Geometry: final body of the model. Coordinates: model frame, mm. Give positions to 0.01 mm unless a question says otherwise; leave off trailing zeros. Write each loop counter-clockwise with the first axis right and the second up, starting at its lowest first coordinate (ties: lowest second). Pieces come first, ordered by that corner, then holes.
Q1. Line query: L1, parallel to Y at x = 0, z = 1; L2, parallel to Y at x = -10, z = 0.45; L3, parallel to X at y = 4.5, z = 2.9 (3 decimals). Output: solid intervals per line, ascending.
Q2. Cut plane D-D on y = -24.13. Return the cut outline in (x, z) (3 decimals), plus the area to 3 significant figures.
Q3. Cut plane B-B on x = 17.78. Return the cut outline in (y, z) (3 decimals).
Q4. Cut plane A-A on y = 12.5. Return the cut outline in (x, z) (3 decimals).
Q5. Pin query (flat end, axial travel): pin 1 (2 mm diameter, centred on x = -55.245, y = -24.13, fed in from -Z). Return the tip coordinate at first contact, or that it passes through.
Q6. Cut plane C-C on y = -6.35. Return the cut outline in (x, z) (3 decimals).
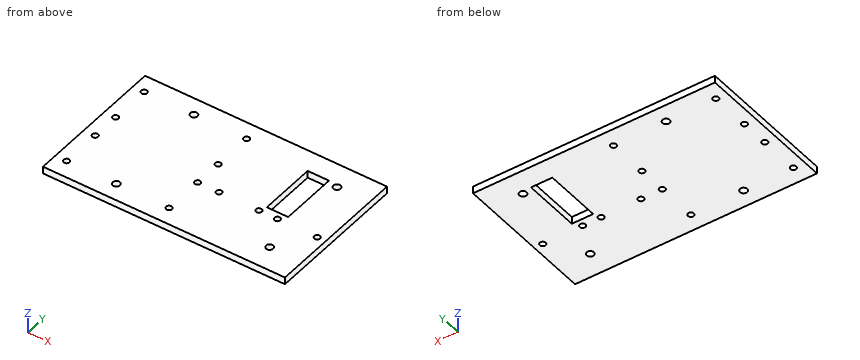
```python
from build123d import *

# Parameters (mm, degrees)
SKETCH1_W               = 95.25
SKETCH1_H               = 63.5
BOSS_EXTRUDE1_DEPTH     = 3.175
SKETCH2_R               = 1.6
CUT_EXTRUDE1_DEPTH      = 58.326117521
CUT_EXTRUDE2_DEPTH      = 58.326117521
CUT_EXTRUDE2_DEPTH_BACK = 58.326117521
SKETCH3_W               = 9.525
SKETCH3_H               = 25.4
SKETCH5_W               = 12.7
SKETCH5_H               = 63.5
BOSS_EXTRUDE2_DEPTH     = 3.175
SKETCH7_R               = 1.3
CUT_EXTRUDE3_DEPTH      = 69.244038201
SKETCH8_R               = 1.29999994
CUT_EXTRUDE4_DEPTH      = 3.175


with BuildPart() as part:
    # Sketch1 → Boss-Extrude1 (new body)
    with BuildSketch(Plane.XY):
        Rectangle(SKETCH1_W, SKETCH1_H)
    extrude(amount=BOSS_EXTRUDE1_DEPTH)

    # Sketch2 → Cut-Extrude1 (cut, through all)
    with BuildSketch(Plane.XY.offset(3.175)):
        with Locations((33.0581, 20.955)):
            Circle(SKETCH2_R)
        with Locations((33.0581, -20.955)):
            Circle(SKETCH2_R)
        with Locations((-33.0581, 24.13)):
            Circle(SKETCH2_R)
        with Locations((-33.0581, -24.13)):
            Circle(SKETCH2_R)
    extrude(amount=-CUT_EXTRUDE1_DEPTH, mode=Mode.SUBTRACT)

    # Sketch3 → Cut-Extrude2 (cut, two sides: drawn at the far end of the back side and taken through both)
    with BuildSketch(Plane.XY.offset(3.175).offset(-CUT_EXTRUDE2_DEPTH_BACK)):
        with Locations((23.8125, 9.525)):
            Rectangle(SKETCH3_W, SKETCH3_H)
    extrude(amount=CUT_EXTRUDE2_DEPTH + CUT_EXTRUDE2_DEPTH_BACK, mode=Mode.SUBTRACT)

    # Sketch5 → Boss-Extrude2 (add)
    with BuildSketch(Plane.XY.offset(3.175)):
        with Locations((-53.975, 0)):
            Rectangle(SKETCH5_W, SKETCH5_H)
    extrude(amount=-BOSS_EXTRUDE2_DEPTH)

    # Sketch7 → Cut-Extrude3 (cut, through all)
    with BuildSketch(Plane.XY.offset(3.175)):
        with Locations((-55.245, 24.13)):
            Circle(SKETCH7_R)
        with Locations((-9.525, 24.13)):
            Circle(SKETCH7_R)
        with Locations((-9.525, 6.35)):
            Circle(SKETCH7_R)
        with Locations((-55.245, 6.35)):
            Circle(SKETCH7_R)
        with Locations((-55.245, -6.35)):
            Circle(SKETCH7_R)
        with Locations((-9.525, -6.35)):
            Circle(SKETCH7_R)
        with Locations((-9.525, -24.13)):
            Circle(SKETCH7_R)
        with Locations((-55.245, -24.13)):
            Circle(SKETCH7_R)
    extrude(amount=-CUT_EXTRUDE3_DEPTH, mode=Mode.SUBTRACT)

    # Sketch8 → Cut-Extrude4 (cut)
    with BuildSketch(Plane.XY.offset(3.175)):
        with Locations((0, -6.35)):
            Circle(SKETCH8_R)
        with Locations((43.815, -6.35)):
            Circle(SKETCH8_R)
        with Locations((17.78, -6.35)):
            Circle(SKETCH8_R)
        with Locations((26.035, -6.35)):
            Circle(SKETCH8_R)
    extrude(amount=-CUT_EXTRUDE4_DEPTH, mode=Mode.SUBTRACT)


solid = part.part
```
Data:
1. L1: y = -31.75 to -7.65, -5.05 to 31.75
1. L2: y = -31.75 to -25.34, -22.92 to -7.56, -5.14 to 5.14, 7.56 to 22.92, 25.34 to 31.75
1. L3: x = -60.325 to 19.05, 28.575 to 47.625
2. outline: (-60.325, 0) - (-56.545, 0) - (-56.545, 3.175) - (-60.325, 3.175) - close; (-53.945, 0) - (-34.658, 0) - (-34.658, 3.175) - (-53.945, 3.175) - close; (-31.458, 0) - (-10.825, 0) - (-10.825, 3.175) - (-31.458, 3.175) - close; (-8.225, 0) - (47.625, 0) - (47.625, 3.175) - (-8.225, 3.175) - close
2. area: 316 mm2
3. outline: (-31.75, 0) - (-7.65, 0) - (-7.65, 3.175) - (-31.75, 3.175) - close; (-5.05, 0) - (31.75, 0) - (31.75, 3.175) - (-5.05, 3.175) - close
4. outline: (-60.325, 0) - (19.05, 0) - (19.05, 3.175) - (-60.325, 3.175) - close; (28.575, 0) - (47.625, 0) - (47.625, 3.175) - (28.575, 3.175) - close
5. pin 1: passes through
6. outline: (-60.325, 0) - (-56.545, 0) - (-56.545, 3.175) - (-60.325, 3.175) - close; (-53.945, 0) - (-10.825, 0) - (-10.825, 3.175) - (-53.945, 3.175) - close; (-8.225, 0) - (-1.3, 0) - (-1.3, 3.175) - (-8.225, 3.175) - close; (1.3, 0) - (16.48, 0) - (16.48, 3.175) - (1.3, 3.175) - close; (19.08, 0) - (24.735, 0) - (24.735, 3.175) - (19.08, 3.175) - close; (27.335, 0) - (42.515, 0) - (42.515, 3.175) - (27.335, 3.175) - close; (45.115, 0) - (47.625, 0) - (47.625, 3.175) - (45.115, 3.175) - close
